Verification items for this drawing (mm, ordinates from the low corner). A direction names the side the tool comes from. Round coordinates to 2 decimals unless told otherwise and drop trailing zeros. Loops run counter-clockwise (first coordinate to the right, second up) from the corner with the lowest first, then second, coordinate; pieces in that order, holes last. Notation, with made-up numbers: (49, 1) - (71, 1) arc R19 cw to (71, 31) - close; hole circle Ø1 at (89, -8.75). An arc over 180 degrees is marked (long way). Put each result on its own line as item: value. Start each with the question number.
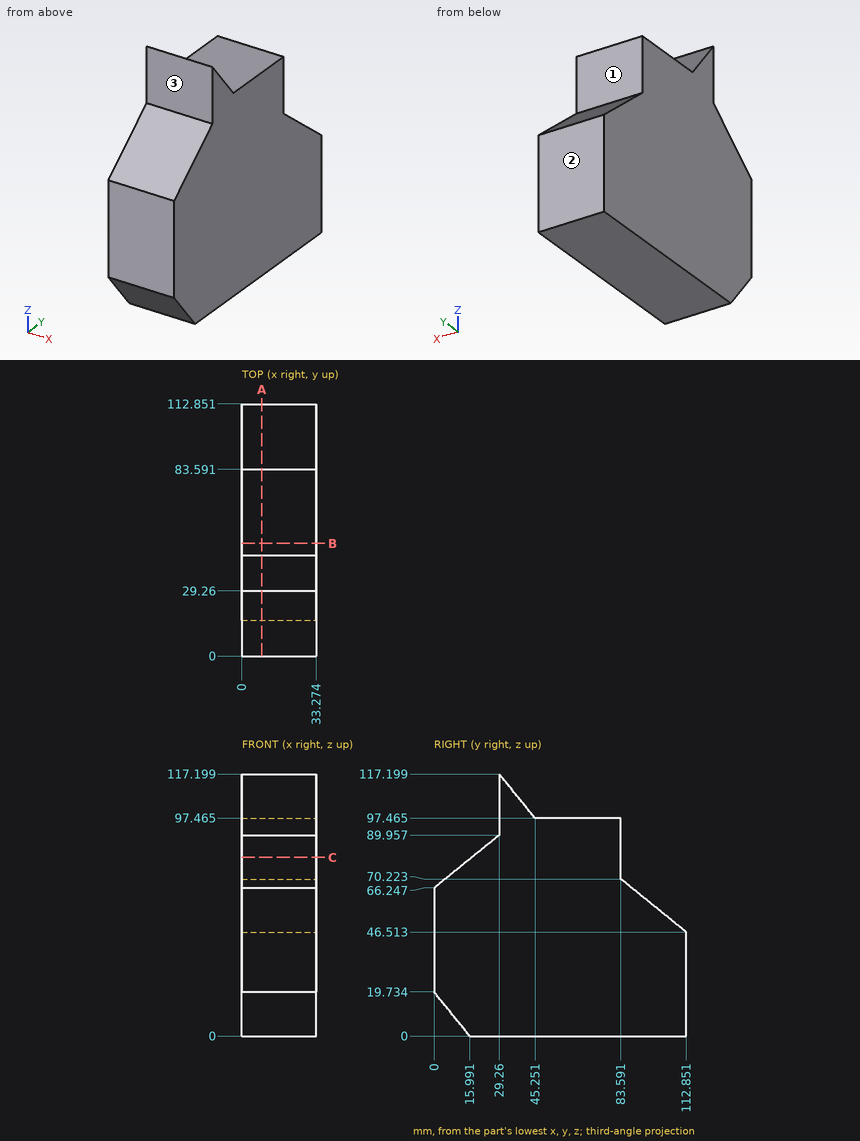
Q1. Material ranges on line 1 (Z direction, x = 25, y = 79.5) (1 decimal); line 2 (Y direction, x = 26.5, z = 92); line 3 (Y direction, x = 31, z = 81) (1 decimal), recorded low to high. Write a range as from..to.
Q2. Depth check by flat-ended pin: pin 1 Ø1 at (x, y) = (21.5, 31.5) entering from +Z; pin 2 Ø3 at (x, z) = (25.5, 84) entering from +Y; pin 3 Ø1 at (x, y) = (8.5, 54.5) entering from +Z (1 decimal). Enter the tip coordinate at first touch or a pass-through.
Q3. Set-up check for the marked faces 1, 2 and 3: record each of +Z, -Z, +X, -X, +Y, -Y from which the full face is reachable in a straight line by a thin tool's end or side.
Q4. Cross-section at C-C on z = 80. Enter the section's corners in (x, y), and give its area (3 significant figures).
Q5. Cross-section at B-B on y = 50.5. Enter the section's corners in (x, z) (1 decimal).
Q6. Cross-section at A-A on x = 9. Enter the section's corners in (y, z) (1 decimal).
Answer list:
1. line 1: z = 0..97.5
1. line 2: y = 29.26..83.59
1. line 3: y = 18.2..83.6
2. pin 1: stops at z = 115.05
2. pin 2: stops at y = 83.59
2. pin 3: stops at z = 97.5
3. face 1: +Z, +X, -X, +Y
3. face 2: +Z, -Z, +X, -X, +Y
3. face 3: +Z, +X, -X, -Y
4. outline: (0, 16.97) - (33.27, 16.97) - (33.27, 83.59) - (0, 83.59) - close
4. area: 2,220 mm2
5. outline: (0, 0) - (33.3, 0) - (33.3, 97.5) - (0, 97.5) - close
6. outline: (0, 19.7) - (16, 0) - (112.9, 0) - (112.9, 46.5) - (83.6, 70.2) - (83.6, 97.5) - (45.3, 97.5) - (29.3, 117.2) - (29.3, 90) - (0, 66.2) - close
